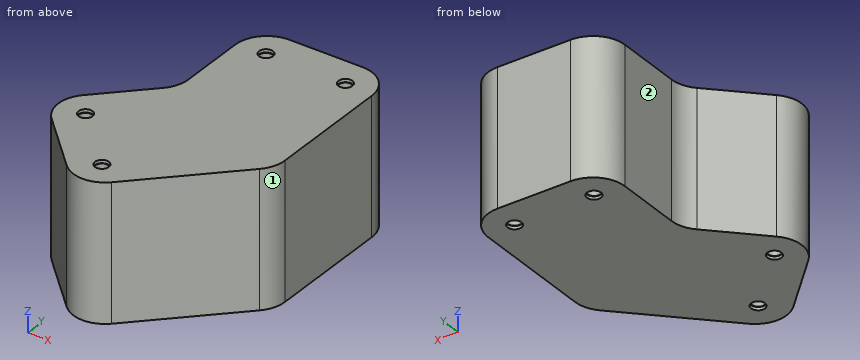
```python
from build123d import *

# Parameters (mm, degrees)
BOSS_EXTRUDE1_DEPTH                          = 42.8
CBORE_FOR_M5_HEX_HEAD_CAP_SCREW1_D           = 4
CBORE_FOR_M5_HEX_HEAD_CAP_SCREW1_DEPTH       = 5.5
CBORE_FOR_M5_HEX_HEAD_CAP_SCREW1_CBORE_D     = 4.4
CBORE_FOR_M5_HEX_HEAD_CAP_SCREW1_CBORE_DEPTH = 1
CBORE_FOR_M5_HEX_HEAD_CAP_SCREW1_TIP         = 1.201721238
CBORE_FOR_M5_HEX_HEAD_CAP_SCREW2_D           = 4
CBORE_FOR_M5_HEX_HEAD_CAP_SCREW2_DEPTH       = 5.5
CBORE_FOR_M5_HEX_HEAD_CAP_SCREW2_CBORE_D     = 4.4
CBORE_FOR_M5_HEX_HEAD_CAP_SCREW2_CBORE_DEPTH = 1
CBORE_FOR_M5_HEX_HEAD_CAP_SCREW2_TIP         = 1.201721238
FILLET1_R                                    = 10


with BuildPart() as part:
    # Sketch3 → Boss-Extrude1 (new body)
    with BuildSketch(Plane.XY):
        Polygon((52.494949366, 117.817279836), (52.494949366, 82.900540957), (27.805086528, 58.210678119), (58.210678119, 27.805086528), (95.494949366, 65.089357775), (95.494949366, 117.817279836), align=None)
    extrude(amount=BOSS_EXTRUDE1_DEPTH)

    # CBORE for M5 Hex Head Cap Screw1
    with Locations(Plane(origin=(0, 0, 0), x_dir=(-1, 0, 0), z_dir=(0, 0, -1))):
        with Locations((-86.494949366, 108.817279836), (-61.494949366, 108.817279836), (-58.210678119, 40.533008589), (-40.533008589, 58.210678119)):
            CounterBoreHole(CBORE_FOR_M5_HEX_HEAD_CAP_SCREW1_D / 2, CBORE_FOR_M5_HEX_HEAD_CAP_SCREW1_CBORE_D / 2, CBORE_FOR_M5_HEX_HEAD_CAP_SCREW1_CBORE_DEPTH, depth=CBORE_FOR_M5_HEX_HEAD_CAP_SCREW1_DEPTH)
            with Locations((0, 0, -(CBORE_FOR_M5_HEX_HEAD_CAP_SCREW1_DEPTH + CBORE_FOR_M5_HEX_HEAD_CAP_SCREW1_TIP / 2))):  # 118° drill point
                Cone(0, CBORE_FOR_M5_HEX_HEAD_CAP_SCREW1_D / 2, CBORE_FOR_M5_HEX_HEAD_CAP_SCREW1_TIP, mode=Mode.SUBTRACT)

    # CBORE for M5 Hex Head Cap Screw2
    with Locations(Plane.XY.offset(42.8)):
        with Locations((61.494949366, 108.817279836), (86.494949366, 108.817279836), (58.210678119, 40.533008589), (40.533008589, 58.210678119)):
            CounterBoreHole(CBORE_FOR_M5_HEX_HEAD_CAP_SCREW2_D / 2, CBORE_FOR_M5_HEX_HEAD_CAP_SCREW2_CBORE_D / 2, CBORE_FOR_M5_HEX_HEAD_CAP_SCREW2_CBORE_DEPTH, depth=CBORE_FOR_M5_HEX_HEAD_CAP_SCREW2_DEPTH)
            with Locations((0, 0, -(CBORE_FOR_M5_HEX_HEAD_CAP_SCREW2_DEPTH + CBORE_FOR_M5_HEX_HEAD_CAP_SCREW2_TIP / 2))):  # 118° drill point
                Cone(0, CBORE_FOR_M5_HEX_HEAD_CAP_SCREW2_D / 2, CBORE_FOR_M5_HEX_HEAD_CAP_SCREW2_TIP, mode=Mode.SUBTRACT)

    # Fillet1
    fillet1_edges = [part.edges().sort_by_distance(p)[0] for p in [
        (95.494949366, 117.817279836, 21.4),
        (95.494949366, 65.089357775, 21.4),
        (58.210678119, 27.805086528, 21.4),
        (27.805086528, 58.210678119, 21.4),
        (52.494949366, 82.900540957, 21.4),
        (52.494949366, 117.817279836, 21.4),
    ]]
    fillet(fillet1_edges, radius=FILLET1_R)


solid = part.part
```
Here's how the part is built. I have some questions about the finished solid (model axes, mm). Face numbers are marked on the shaded views. A direction names the side the tool comes from. Give positions to 0.01 mm unless a question says otherwise; leave off trailing zeros. Write each loop counter-clockwise with the first axis right and the second up, starting at its lowest first coordinate (ties: lowest second). Pieces come first, ordered by that corner, then holes.
(1) Imagine slicing it at D-D, the plane y = 84. Write out the boundary of the cut face in (x, z), and give its area (3 significant figures).
Output values:
outline: (52.02, 0) - (95.49, 0) - (95.49, 42.8) - (52.02, 42.8) - close
area: 1,860 mm2
(2) Imagine slicing it at C-C, the plane x = 72.5. Write out the boundary of the cut face in (y, z), and give its area (3 significant figures).
Output values:
outline: (42.09, 0) - (117.82, 0) - (117.82, 42.8) - (42.09, 42.8) - close
area: 3,240 mm2
(3) Imagine slicing it at B-B, the plane z = 4. Write out the boundary of the cut face in (x, y).
Output values:
outline: (34.88, 51.14) - (51.14, 34.88) arc R10 ccw to (65.28, 34.88) - (92.57, 62.16) arc R10 ccw to (95.49, 69.23) - (95.49, 107.82) arc R10 ccw to (85.49, 117.82) - (62.49, 117.82) arc R10 ccw to (52.49, 107.82) - (52.49, 87.04) arc R10 cw to (49.57, 79.97) - (34.88, 65.28) arc R10 ccw to start; hole circle Ø4 at (40.53, 58.21); hole circle Ø4 at (58.21, 40.53); hole circle Ø4 at (61.49, 108.82); hole circle Ø4 at (86.49, 108.82)
(4) If I drill on L1, parallel to X at y = 107.5, z = 2; L2, parallel to X at y = 102, z = 31; L3, parallel to X at y = 82, z = 17, over which ranges is the centre line in solid material (lowest first)?
Output values:
L1: x = 52.49 to 59.99, 63 to 84.99, 88 to 95.49
L2: x = 52.49 to 95.49
L3: x = 51.13 to 95.49
(5) Will these pins go through, and if not, where does the flat tip stop? pin 1 (2 mm diameter, centred on x = 87, y = 109, fed in from +Z); pin 2 (2 mm diameter, centred on x = 39.5, y = 58.5, fed in from -Z); pin 3 (2.5 mm diameter, centred on x = 58.21, y = 40.53, fed in from +Z); pin 4 (5 mm diameter, centred on x = 40, y = 59, fed in from +Z).
Output values:
pin 1: stops at z = 37.02
pin 2: stops at z = 1
pin 3: stops at z = 36.85
pin 4: stops at z = 42.8
(6) Imagine slicing it at A-A, the plane z = 18. Write out the boundary of the cut face in (x, y), and give its area (3 significant figures).
Output values:
outline: (34.88, 51.14) - (51.14, 34.88) arc R10 ccw to (65.28, 34.88) - (92.57, 62.16) arc R10 ccw to (95.49, 69.23) - (95.49, 107.82) arc R10 ccw to (85.49, 117.82) - (62.49, 117.82) arc R10 ccw to (52.49, 107.82) - (52.49, 87.04) arc R10 cw to (49.57, 79.97) - (34.88, 65.28) arc R10 ccw to start
area: 3,680 mm2
(7) On a 3-axis mill with a long thin cutter (end or side, diameter ignored), from which of +Z, -Z, +X, -X, +Y, -Y can I reach the whole of each face in a straight line? I mean the marked faces 1 and 2. Say none if no direction works.
Output values:
face 1: +Z, -Z, +X, -Y
face 2: +Z, -Z, -X, +Y
